Autodesk Inventor part; units mm, degrees
ref_plane "YZ Plane" through (0, 0, 0) normal (1, 0, 0) x (0, 1, 0)
ref_plane "XZ Plane" through (0, 0, 0) normal (0, 1, 0) x (-1, 0, 0)
ref_plane "XY Plane" through (0, 0, 0) normal (0, 0, 1) x (1, 0, 0)
sketch "Skizze1" plane through (0, 0, 0) normal (0, 0, 1) x (1, 0, 0)
  line L0 (0, 0) -> (0, 2)
  line L1 (0, 2) -> (-17, 2)
  line L2 (-17, 2) -> (-17, 10)
  line L3 (-17, 10) -> (-31, 10)
  line L4 (-31, 10) -> (-31, 0)
  line L5 (-31, 0) -> (0, 0)
  dimension "d0" = 17
  dimension "d1" = 2
  dimension "d2" = 14
  dimension "d3" = 10
extrude "Extrusion1" add sketch "Skizze1" along normal mid plane 19
sketch "Skizze2" plane through (-31, 10, 9.5) normal (0, 1, 0) x (1, 0, 0)
  circle A0 centre (7, 5) radius 2.5
  line L0 (14, 0) -> (0, 0)
  point P0 (31, 9.5)
  point P1 (7, 0)
  dimension "d6" = 5
  dimension "d7" = 5
extrude "Extrusion2" add sketch "Skizze2" along normal blind 3
sketch "Skizze3" plane through (-24, 13, 4.5) normal (0, 1, 0) x (1, 0, 0)
  circle A0 centre (0, 0) radius 2
  point P0 (24, 4.5)
  dimension "d10" = 4
extrude "Extrusion3" cut sketch "Skizze3" against normal through all
sketch "Skizze4" plane through (-31, 10, 9.5) normal (0, 1, 0) x (1, 0, 0)
  line L0 (5.5, 14.5) -> (8.5, 14.5)
  line L1 (8.5, 14.5) -> (8.5, 16)
  line L2 (8.5, 16) -> (5.5, 16)
  line L3 (5.5, 16) -> (5.5, 14.5)
  line L4 (0, 19) -> (14, 19)
  point P0 (31, 9.5)
  point P1 (7, 16)
  point P2 (7, 19)
  dimension "d13" = 1.5
  dimension "d14" = 3
  dimension "d15" = 3
extrude "Extrusion4" cut sketch "Skizze4" against normal through all
sketch "Skizze5" plane through (-31, 10, 9.5) normal (0, 1, 0) x (1, 0, 0)
  line L0 (5.5, 16) -> (8.5, 16)
  line L1 (5, 14) -> (9, 14)
  line L2 (9, 14) -> (9, 16.5)
  line L3 (9, 16.5) -> (5, 16.5)
  line L4 (5, 16.5) -> (5, 14)
  line L5 (5.5, 14.5) -> (5.5, 16)
  line L6 (8.5, 16) -> (8.5, 14.5)
  line L7 (8.5, 14.5) -> (5.5, 14.5)
  point P0 (31, 9.5)
  point P1 (5, 15.25)
  point P2 (5.5, 15.25)
  point P3 (7, 14)
  point P4 (7, 16)
  dimension "d18" = 0.5
  dimension "d19" = 0.5
extrude "Extrusion5" add sketch "Skizze5" along normal blind 2
sketch "Skizze6" plane through (-31, 10, 9.5) normal (0, 1, 0) x (1, 0, 0)
  line L0 (0, 19) -> (0, 0)
  line L1 (0, 19) -> (14, 19)
  line L2 (14, 19) -> (14, 0)
  line L3 (14, 0) -> (0, 0)
  line L4 (1, 1) -> (13, 1)
  line L5 (13, 1) -> (13, 18)
  line L6 (13, 18) -> (1, 18)
  line L7 (1, 18) -> (1, 1)
  point P0 (31, 9.5)
  point P1 (1, 9.5)
  point P2 (0, 9.5)
  point P3 (7, 18)
  point P4 (7, 19)
  dimension "d22" = 1
  dimension "d23" = 1
extrude "Extrusion6" add sketch "Skizze6" along normal blind 1
sketch "Skizze7" plane through (-17, 2, 9.5) normal (0, 1, 0) x (1, 0, 0)
  line L0 (17, 19) -> (17, 0)
  line L1 (17, 19) -> (17, 14)
  line L2 (17, 14) -> (13.5, 14)
  line L3 (17, 0) -> (17, 5)
  line L4 (17, 5) -> (13.5, 5)
  point P0 (17, 9.5)
  dimension "d26" = 5
  dimension "d27" = 3.5
  dimension "d28" = 5
  dimension "d29" = 3.5
hole "Bohrung1" at (-3.5, 2, 4.5) at (-3.5, 2, -4.5) direction (0, -1, 0) diameter 4 depth 50 tip angle 118
properties part number "Deck_neu"
Source: CAD feature listing. Evaluate the final solid. Frame: model axes, mm. A direction names the side the tool comes from. Round coordinates to 2 decimals unless told otherwise and drop trailing zeros. Loops run counter-clockwise (first coordinate to the right, second up) from the corner with the lowest first, then second, coordinate; pieces in that order, holes last.
1. Section query D-D on y = 5.75. Output: boundary loops of the cut face in (x, z).
2. Contact query for flat-ended pins moving along their axis: pin 1 (5 mm diameter, centred on y = 6, z = 6, fed in from +X); pin 2 (1.6 mm diameter, centred on x = -23.5, y = 11.5, fed in from -Z); pin 3 (4.5 mm diameter, centred on x = -3.5, z = 4.5, fed in from +Y); pin 4 (1.2 mm diameter, centred on x = -24.5, z = -6, fed in from +Y). Output: stop coordinate, or through.
3. Mould query, pull axis Z, two halves, no side actions, for faces 4 (the flat face through (-24, 11, -7)), 5 (the flat face through (-22, 4, 9.5)), 6 (the flat face through (-16, 0, 0)). Classes: released by +Z, released by -Z, zero draft, split by the parting line, or undercut.
4. Section query C-C on z = 4.5. Output: boundary loops of the cut face in (x, y), and give its area (3 significant figures).
5. Access query for faces 1 (the flat face through (-30, 10.5, -0.1)), 2 (the flat face through (-25.5, 6, -6)), 3 (the flat face through (-8, 2, 0)). Directions: +Z, -Z, +X, -X, +Y, -Y. A direction counts if a zero-diameter tool reaches every point of the face in a straight line with its end or side. Return the directions, or none.
6. Section query A-A on y = 10.5. Output: boundary loops of the cut face in (x, z), and give its area (3 significant figures).
7. Section query B-B on x = -24. Output: boundary loops of the cut face in (y, z).
8. Ray query, L1, parallel to Z at x = -3.5, y = 0.7; L2, parallel to Z at x = -24, y = 6.25; L3, parallel to X at y = 8.25, z = 4.5. Return the intervals inside material, ascending.
Answers below:
1. outline: (-31, -9.5) - (-17, -9.5) - (-17, 9.5) - (-31, 9.5) - close; hole circle Ø4 at (-24, 4.5); hole (-25.5, -6.5) - (-22.5, -6.5) - (-22.5, -5) - (-25.5, -5) - close
2. pin 1: stops at x = -17
2. pin 2: stops at z = -9.5
2. pin 3: stops at y = 2
2. pin 4: stops at y = 12
3. face 4: undercut
3. face 5: released by +Z
3. face 6: zero draft
4. outline: (-31, 0) - (-26, 0) - (-26, 13) - (-26.5, 13) - (-26.5, 10) - (-30, 10) - (-30, 11) - (-31, 11) - close; (-22, 0) - (-5.5, 0) - (-5.5, 2) - (-17, 2) - (-17, 11) - (-18, 11) - (-18, 10) - (-21.5, 10) - (-21.5, 13) - (-22, 13) - close; (-1.5, 0) - (0, 0) - (0, 2) - (-1.5, 2) - close
4. area: 131 mm2
5. face 1: +Y
5. face 2: +Y, -Y
5. face 3: +Z, -Z, +X, +Y
6. outline: (-31, -9.5) - (-17, -9.5) - (-17, 9.5) - (-31, 9.5) - close; circle Ø5 at (-24, 4.5); (-26, -7) - (-22, -7) - (-22, -4.5) - (-26, -4.5) - close; hole (-30, -8.5) - (-18, -8.5) - (-18, 8.5) - (-30, 8.5) - close; hole circle Ø4 at (-24, 4.5); hole (-25.5, -6.5) - (-22.5, -6.5) - (-22.5, -5) - (-25.5, -5) - close
6. area: 74.6 mm2
7. outline: (0, -9.5) - (11, -9.5) - (11, -8.5) - (10, -8.5) - (10, -7) - (12, -7) - (12, -6.5) - (0, -6.5) - close; (0, -5) - (12, -5) - (12, -4.5) - (10, -4.5) - (10, 2) - (13, 2) - (13, 2.5) - (0, 2.5) - close; (0, 6.5) - (13, 6.5) - (13, 7) - (10, 7) - (10, 8.5) - (11, 8.5) - (11, 9.5) - (0, 9.5) - close
8. L1: z = -9.5 to -6.5, -2.5 to 2.5, 6.5 to 9.5
8. L2: z = -9.5 to -6.5, -5 to 2.5, 6.5 to 9.5
8. L3: x = -31 to -26, -22 to -17
